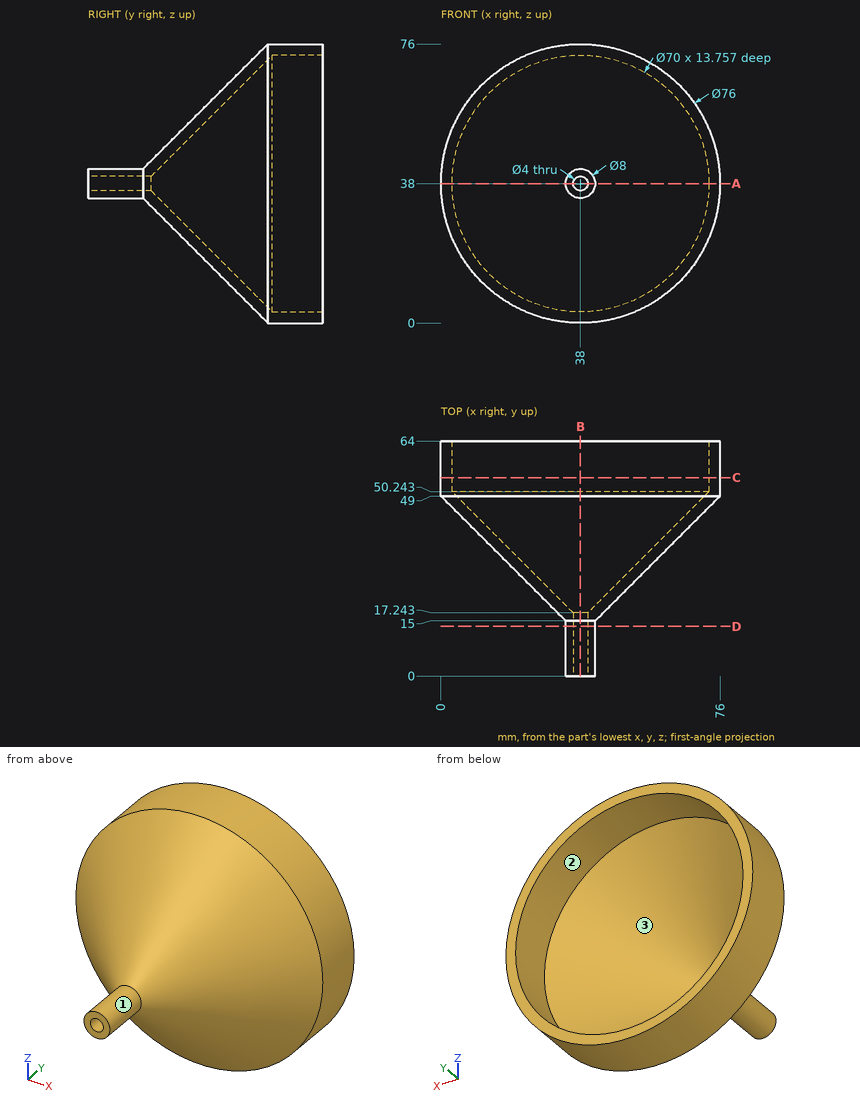
Here's the drawing with two shaded views (mm, measured from the low corner). I have some questions. Give positions to 0.01 mm unless a question says otherwise; leave off trailing zeros. Order: outer loops, then holes, each group sorted by start corner. A loop starts at its lowest first (then second) coordinate and runs counter-clockwise, first axis right, second up. Notation, with made-up numbers: (-3, -3.5) - (6, -3.5) arc R31 ccw to (6, 23.5) - close; hole circle Ø11 at (43.5, 23.5). An arc over 180 degrees is marked (long way). Write each question's results on one line, items separated by ' | '.
1) Suppose I cut it at B-B, the plane x = 38. Write out the boundary of the cut face in (y, z).
Final values:
outline: (0, 34) - (15, 34) - (49, 0) - (64, 0) - (64, 3) - (50.24, 3) - (17.24, 36) - (0, 36) - close; (0, 40) - (17.24, 40) - (50.24, 73) - (64, 73) - (64, 76) - (49, 76) - (15, 42) - (0, 42) - close
2) Suppose I cut it at C-C, the plane y = 54. Write out the boundary of the cut face in (x, z), then the cut area to 3 significant figures.
Final values:
outline: circle Ø76 at (38, 38); hole circle Ø70 at (38, 38) | area: 688 mm^2
3) Suppose I cut it at D-D, the plane y = 13.5. Write out the boundary of the cut face in (x, z), then the cut area to 3 significant figures.
Final values:
outline: circle Ø8 at (38, 38); hole circle Ø4 at (38, 38) | area: 37.7 mm^2
4) Suppose I cut it at A-A, the plane z = 38. Write out the boundary of the cut face in (x, y), then the cut area to 3 significant figures.
Final values:
outline: (0, 49) - (34, 15) - (34, 0) - (36, 0) - (36, 17.24) - (3, 50.24) - (3, 64) - (0, 64) - close; (40, 0) - (42, 0) - (42, 15) - (76, 49) - (76, 64) - (73, 64) - (73, 50.24) - (40, 17.24) - close | area: 435 mm^2
5) Please list where these lines run through material, in increasing order: line 1 along X through (y, z) = (4, 38); line 2 along Z through (x, y) = (38, 58). Write a range as [from, to].
Final values:
line 1: x = [34, 36], [40, 42] | line 2: z = [0, 3], [73, 76]
6) I'm going to push flat-ended pins straight in: pin 1 Ø8 at (x, z) = (14.5, 48) entering from +Y; pin 2 Ø10 at (x, y) = (19, 33) entering from +Z (1 decimal); pin 3 Ø1.5 at (x, y) = (33, 12) entering from -Z; pin 4 Ø3 at (x, z) = (18, 25) entering from -Y (1 decimal). Where does each tip first touch, or does it pass through?
Final values:
pin 1: stops at y = 44.78 | pin 2: stops at z = 58.5 | pin 3: passes through | pin 4: stops at y = 33.4
7) If we mould it in two halves opening along Z, with no side actions, what happens to the marked faces 1, 2 and 3? For each: pulls with the +Z half, pulls with the -Z half, needs draft (parallel to the pull), parting line crosses it, or undercut.
Final values:
face 1: parting line crosses it | face 2: undercut | face 3: undercut
